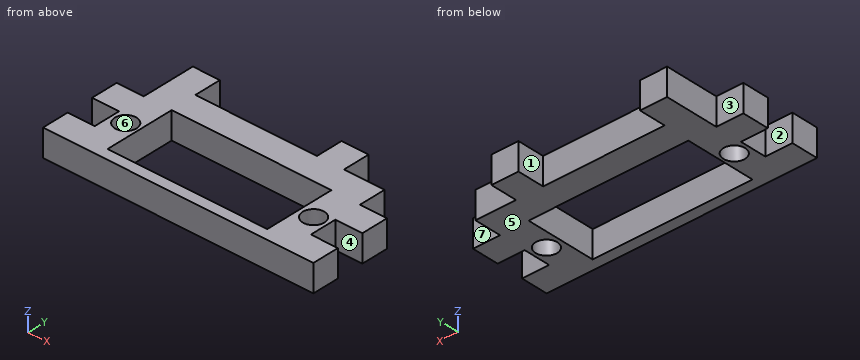
```python
from build123d import *

# Parameters (mm, degrees)
ESQUISSE1_W             = 25
ESQUISSE1_H             = 25
BOSS_EXTRU_1_DEPTH      = 5
ESQUISSE3_W             = 5
ESQUISSE3_H             = 5
ENL_V_MAT_EXTRU_1_DEPTH = 5
ESQUISSE4_R             = 2
ESQUISSE4_W             = 29.55
ESQUISSE4_H             = 13.05
ENL_V_MAT_EXTRU_2_DEPTH = 5
ESQUISSE5_W             = 5
ESQUISSE5_H             = 5
BOSS_EXTRU_2_DEPTH      = 5


with BuildPart() as part:
    # Esquisse1 → Boss.-Extru.1 (new body)
    with BuildSketch(Plane.XY):
        with Locations((-53.521610088, -25.407575758)):
            Rectangle(ESQUISSE1_W, ESQUISSE1_H)
    boss_extru_1 = extrude(amount=BOSS_EXTRU_1_DEPTH)

    # Esquisse3 → Enlèv. mat.-Extru.1 (cut)
    with BuildSketch(Plane(origin=(0, 0, 0), x_dir=(-1, 0, 0), z_dir=(0, 0, -1))):
        Polygon((66.021610088, -12.907575758), (66.021610088, -17.907575758), (46.021610088, -17.907575758), (46.021610088, -22.907575758), (41.021610088, -22.907575758), (41.021610088, -12.907575758), align=None)
        with Locations((43.521610088, -30.407575758)):
            Rectangle(ESQUISSE3_W, ESQUISSE3_H)
    enl_v_mat_extru_1 = extrude(amount=-ENL_V_MAT_EXTRU_1_DEPTH, mode=Mode.SUBTRACT)

    # Symétrie1: Boss.-Extru.1, Enlèv. mat.-Extru.1 across plane
    add(boss_extru_1.mirror(Plane(origin=(-66.021610088, -12.907575758, 5), x_dir=(0, 0, 1), z_dir=(1, 0, 0))))
    add(enl_v_mat_extru_1.mirror(Plane(origin=(-66.021610088, -12.907575758, 5), x_dir=(0, 0, 1), z_dir=(1, 0, 0))), mode=Mode.SUBTRACT)

    # Esquisse4 → Enlèv. mat.-Extru.2 (cut)
    with BuildSketch(Plane(origin=(0, 0, 0), x_dir=(-1, 0, 0), z_dir=(0, 0, -1))):
        with Locations((83.396610088, -29.457575758)):
            Circle(ESQUISSE4_R)
        with Locations((48.646610088, -29.457575758)):
            Circle(ESQUISSE4_R)
        with Locations((66.121610088, -29.382575758)):
            Rectangle(ESQUISSE4_W, ESQUISSE4_H)
    extrude(amount=-ENL_V_MAT_EXTRU_2_DEPTH, mode=Mode.SUBTRACT)

    # Esquisse5 → Boss.-Extru.2 (add)
    with BuildSketch(Plane(origin=(0, -17.907575758, 0), x_dir=(1, 0, 0), z_dir=(0, 1, 0))):
        with Locations((-83.521610088, -2.5)):
            Rectangle(ESQUISSE5_W, ESQUISSE5_H)
        with Locations((-56.021610088, -2.5)):
            Rectangle(ESQUISSE5_W, ESQUISSE5_H)
    extrude(amount=BOSS_EXTRU_2_DEPTH)


solid = part.part
```
Could you check a few things on this model? Use its own coordinates, in mm. Face numbers are marked on the shaded views. A direction names the side the tool comes from. Coordinates: 2 decimals unless noted, no trailing zeros. Write each loop counter-clockwise with the first axis right and the second up, starting at its lowest first coordinate (ties: lowest second). Pieces come first, ordered by that corner, then holes. Notation, with made-up numbers: (-22.75, 43) - (16.25, 43) arc R6 ccw to (16.25, 54) - close; hole circle Ø9 at (68, -24). An arc over 180 degrees is marked (long way). Use a Markdown table: item, result.
Q1. Thinking about a two-plate mould opening in Y: for the marked faces 5, 6 and 7, which applies, +Y half, -Y half, draft (parallel to the pull), parting line (faces both ways), or undercut?
Geometry check:
| item | result |
|---|---|
| face 5 | draft |
| face 6 | undercut |
| face 7 | +Y half |
Q2. Imagine slicing it at D-D (z = 2.75). List the corners of the cut face in (x, y) for me.
Geometry check:
| item | result |
|---|---|
| outline | (-91.02, -37.91) - (-41.02, -37.91) - (-41.02, -32.91) - (-46.02, -32.91) - (-46.02, -27.91) - (-41.02, -27.91) - (-41.02, -22.91) - (-46.02, -22.91) - (-46.02, -17.91) - (-53.52, -17.91) - (-53.52, -12.91) - (-58.52, -12.91) - (-58.52, -17.91) - (-81.02, -17.91) - (-81.02, -12.91) - (-86.02, -12.91) - (-86.02, -22.91) - (-91.02, -22.91) - (-91.02, -27.91) - (-86.02, -27.91) - (-86.02, -32.91) - (-91.02, -32.91) - close; hole circle Ø4 at (-83.4, -29.46); hole (-80.9, -35.91) - (-51.35, -35.91) - (-51.35, -22.86) - (-80.9, -22.86) - close; hole circle Ø4 at (-48.65, -29.46) |
Q3. Imagine slicing it at B-B (y = -17). List the corners of the cut face in (x, z) for me, and give its area (3 significant figures).
Geometry check:
| item | result |
|---|---|
| outline | (-86.02, 0) - (-81.02, 0) - (-81.02, 5) - (-86.02, 5) - close; (-58.52, 0) - (-53.52, 0) - (-53.52, 5) - (-58.52, 5) - close |
| area | 50.0 mm2 |
Q4. I'm going to push flat-ended pins straight in: pin 1 Ø1.5 at (y, z) = (-31, 2.5) entering from -X; pin 2 Ø1 at (y, z) = (-30.5, 2.5) entering from +X; pin 3 Ø3 at (x, y) = (-65.5, -33.5) entering from -Z; pin 4 Ø2.5 at (x, z) = (-89.5, 2.5) entering from +Y. Where does each tip first touch, or does it pass through?
Geometry check:
| item | result |
|---|---|
| pin 1 | stops at x = -86.02 |
| pin 2 | stops at x = -46.02 |
| pin 3 | passes through |
| pin 4 | stops at y = -22.91 |
Q5. Please list where these lines run through material, in increasing order: L1, parallel to Y at x = -62, z = 0.65; L2, parallel to X at y = -34, z = 1.5; L3, parallel to X at y = -17, z = 3.85.
Geometry check:
| item | result |
|---|---|
| L1 | y = -37.91 to -35.91, -22.86 to -17.91 |
| L2 | x = -91.02 to -80.9, -51.35 to -41.02 |
| L3 | x = -86.02 to -81.02, -58.52 to -53.52 |
Q6. Which directions (+Z, -Z, +X, -X, +Y, -Y) give clear straight access to the entire face, cutting with the end or side of a thin tool? Please do the marked faces 1, 2, 3 and 4.
Geometry check:
| item | result |
|---|---|
| face 1 | +Z, -Z, +Y |
| face 2 | +Z, -Z, -X |
| face 3 | +Z, -Z, -X, +Y |
| face 4 | +Z, -Z, +X |
Q7. Imagine slicing it at A-A (x = -61). List the corners of the cut face in (y, z) for me, and give its area (4 significant figures).
Geometry check:
| item | result |
|---|---|
| outline | (-37.91, 0) - (-35.91, 0) - (-35.91, 5) - (-37.91, 5) - close; (-22.86, 0) - (-17.91, 0) - (-17.91, 5) - (-22.86, 5) - close |
| area | 34.75 mm2 |
Q8. Imagine slicing it at C-C (y = -30.25). List the corners of the cut face in (x, z) for me.
Geometry check:
| item | result |
|---|---|
| outline | (-86.02, 0) - (-85.23, 0) - (-85.23, 5) - (-86.02, 5) - close; (-81.56, 0) - (-80.9, 0) - (-80.9, 5) - (-81.56, 5) - close; (-51.35, 0) - (-50.48, 0) - (-50.48, 5) - (-51.35, 5) - close; (-46.81, 0) - (-46.02, 0) - (-46.02, 5) - (-46.81, 5) - close |
